Verification items for the finished model (mm, model axes). Face numbers are marked on the shaded views. A direction names the side the tool comes from. Coordinates: 2 decimals unless noted, no trailing zeros. Write each loop counter-clockwise with the first axis right and the second up, starting at its lowest first coordinate (ties: lowest second). Pieces come first, ordered by that corner, then holes. Notation, with made-up numbers: (-15, -21) -> (18, -21) arc R22 cw to (18, -4) -> close; hole circle Ø5 at (-35.5, 48.5). An arc over 180 degrees is marked (long way). Answer in a Markdown table with one row per item.
Autodesk Fusion 360 part; units mm, degrees
sketch "Çizim1" plane through (0, 0, 0) normal (0, 0, 1) x (1, 0, 0)
  line L0 (52.5, 65) -> (-52.5, 65)
  line L1 (-52.5, 65) -> (-52.5, -65)
  line L2 (-52.5, -65) -> (52.5, -65)
  line L3 (52.5, -65) -> (52.5, 65)
  line L4 (52.5, 65) -> (-52.5, -65) construction
  line L5 (-52.5, 65) -> (52.5, -65) construction
  dimension "d1" = 105
  dimension "d2" = 130
extrude "Ekstrüzyon1" add sketch "Çizim1" against normal blind 5
sketch "Çizim2" plane through (0, 0, 0) normal (0, 0, 1) x (-1, 0, 0)
  line L0 (-52.5, 65) -> (-52.5, -65)
  line L1 (-52.5, -65) -> (52.5, -65)
  line L2 (52.5, -65) -> (52.5, 65)
  line L3 (52.5, 65) -> (-52.5, 65)
  line L4 (47.5, 60) -> (-47.5, 60)
  line L5 (-47.5, 60) -> (-47.5, -60)
  line L6 (-47.5, -60) -> (47.5, -60)
  line L7 (47.5, -60) -> (47.5, 60)
  dimension "d5" = -5
extrude "Ekstrüzyon2" add sketch "Çizim2" along normal blind 30
extrude "Ekstrüzyon3" add 1 faces at (-47.5, 20, 10) along direction (1, 0, 0) blind 2.5
extrude "Ekstrüzyon4" add 1 faces at (47.5, -20, 10) along direction (-1, 0, 0) blind 2.5
extrude "Ekstrüzyon5" add 1 faces at (-50, 20, 30) along direction (0, 0, 1) blind 20
extrude "Ekstrüzyon6" add 1 faces at (-17.5, -65, 13.3333) along direction (0, -1, 0) blind 2
extrude "Ekstrüzyon7" add 1 faces at (-17.5, 65, 31.6667) along direction (0, 1, 0) blind 2
sketch "Çizim4" plane through (52.5, 0, 0) normal (1, 0, 0) x (0, 1, 0)
  line L0 (-67, -5) -> (67, -5)
  line L1 (67, -5) -> (67, 50)
  line L2 (67, 50) -> (-67, 50)
  line L3 (-67, 50) -> (-67, -5)
  circle A0 centre (-61, 40.25) radius 1.3
  line L4 (0, 50) -> (0, -5)
  circle A1 centre (61, 40.25) radius 1.3
  dimension "d18" = 2.6
  dimension "d19" = 9.75
  dimension "d20" = 6
extrude "Ekstrüzyon8" cut sketch "Çizim4" against normal blind 7.5 contours A0 | A1
extrude "Ekstrüzyon9" add 1 faces at (-15, 60, 29.8064) along direction (0, -1, 0) blind 5
extrude "Ekstrüzyon10" add 1 faces at (-15, -60, 29.8064) along direction (0, 1, 0) blind 5
mirror "Ayna1" about plane through (0, 0, 0) normal (1, 0, 0) of "Ekstrüzyon8"
sketch "Çizim5" plane through (-52.5, 0, 0) normal (-1, 0, 0) x (0, -1, 0)
  circle A0 centre (61, 40.25) radius 1.3
  circle A1 centre (-61, 40.25) radius 1.3
  line L0 (-67, -5) -> (67, -5)
  line L1 (67, -5) -> (67, 50)
  line L2 (67, 50) -> (-67, 50)
  line L3 (-67, 50) -> (-67, -5)
  line L4 (-55, 40) -> (-55, 25)
  line L5 (55, 40) -> (55, 25)
  line L6 (-55, 40) -> (55, 40)
  line L7 (55, 40) -> (55, 25)
  line L8 (55, 25) -> (-55, 25)
  line L9 (-55, 25) -> (-55, 40)
  dimension "d29" = 12
  dimension "d30" = 15
  dimension "d31" = 15
  dimension "d32" = 12
  dimension "d33" = 10
extrude "Ekstrüzyon11" cut sketch "Çizim5" against normal blind 105 contours L4 L5 L6 L7 L8 L9
sketch "Çizim6" plane through (-52.5, 0, 0) normal (-1, 0, 0) x (0, -1, 0)
  line L0 (55, 40) -> (55, 25)
  line L1 (55, 25) -> (-55, 25)
  line L2 (-55, 25) -> (-55, 40)
  line L3 (-55, 40) -> (55, 40)
  circle A0 centre (61, 40.25) radius 1.3
  circle A1 centre (-61, 40.25) radius 1.3
  line L4 (-67, -5) -> (67, -5)
  line L5 (67, -5) -> (67, 50)
  line L6 (67, 50) -> (-67, 50)
  line L7 (-67, 50) -> (-67, -5)
  line L8 (55, 25) -> (55, -5)
  line L9 (-55, 25) -> (-55, -5)
  line L10 (-55, 10) -> (55, 10)
  line L11 (-55, 20) -> (55, 20)
  line L12 (55, 20) -> (55, 0)
  line L13 (55, 0) -> (-55, 0)
  line L14 (-55, 0) -> (-55, 20)
extrude "Ekstrüzyon12" cut sketch "Çizim6" against normal blind 105 contours L8 L9 L10 L11 L12 L14 | L8 L9 L10 L12 L13 L14
sketch "Çizim7" plane through (0, 67, 0) normal (0, 1, 0) x (-1, 0, 0)
  line L0 (-52.5, 50) -> (-52.5, -5)
  line L1 (-52.5, -5) -> (52.5, -5)
  line L2 (52.5, -5) -> (52.5, 50)
  line L3 (52.5, 50) -> (-52.5, 50)
  line L4 (-45, 50) -> (-45, -5)
  line L5 (45, 50) -> (45, -5)
  line L6 (-45, 45) -> (45, 45)
  line L7 (45, 45) -> (45, 0)
  line L8 (45, 0) -> (-45, 0)
  line L9 (-45, 0) -> (-45, 45)
  dimension "d38" = 7.5
  dimension "d39" = 7.5
extrude "Ekstrüzyon13" cut sketch "Çizim7" against normal blind 134 contours L4 L5 L6 L7 L8 L9
sketch "Çizim8" plane through (0, 0, -5) normal (0, 0, -1) x (1, 0, 0)
  line L0 (52.5, -67) -> (52.5, 67)
  line L1 (52.5, 67) -> (-52.5, 67)
  line L2 (-52.5, 67) -> (-52.5, -67)
  line L3 (-52.5, -67) -> (52.5, -67)
  line L4 (5.5, -35.9) -> (-5.5, -35.9)
  line L5 (-5.5, -35.9) -> (-5.5, -56.1)
  line L6 (-5.5, -56.1) -> (5.5, -56.1)
  line L7 (5.5, -56.1) -> (5.5, -35.9)
  line L8 (0, -35.9) -> (0, -56.1)
  circle A0 centre (11.6, -31.8) radius 1.3
  circle A1 centre (11.6, -60.2) radius 1.3
  line L9 (11.6, -31.8) -> (11.6, -33.1)
  line L10 (11.6, -31.8) -> (11.6, -33.1)
  line L11 (11.6, -58.9) -> (11.6, -60.2)
  line L12 (11.6, -31.8) -> (11.6, -60.2)
  line L13 (11.6, -46) -> (5.5, -46)
  point P0 (5.5, -46)
  dimension "d42" = 11
  dimension "d43" = 20.2
  dimension "d44" = 10.9
  dimension "d45" = 28.4
  dimension "d46" = 2.6
  dimension "d47" = 2.6
  dimension "d48" = 6.1
extrude "Ekstrüzyon14" cut sketch "Çizim8" against normal blind 5 contours L4 L6 L7 L8 | A0 | A1 | L4 L5 L6 L8
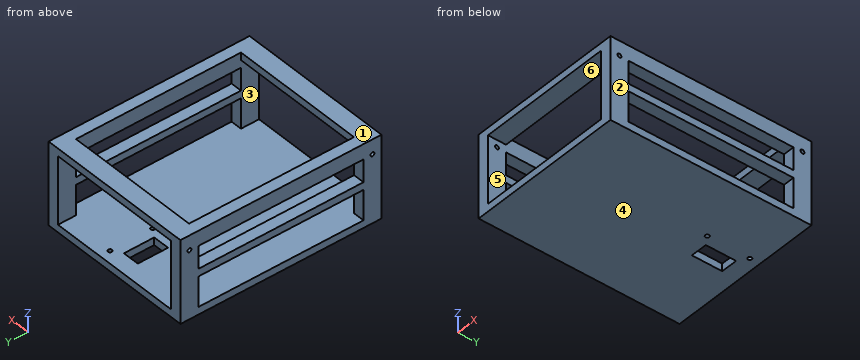
1. Depth check by flat-ended pin: P1, Ø4, axis at x = 27, y = 37.5, coming from the +Z side; P2, Ø3.5, axis at y = 61, z = 40.25, coming from the -X side. Enter the tip coordinate at first touch or a pass-through.
Geometry says:
| item | result |
|---|---|
| P1 | z = 0 |
| P2 | x = -52.5 |
2. Thickness scan on line 1 (X direction, y = -55.5, z = 36.5); line 2 (Y direction, x = 30, z = 46.5); line 3 (Z direction, x = 50, y = -61). Record the ranges inside material, lowest first. Write a range as from..to.
Geometry says:
| item | result |
|---|---|
| line 1 | -52.5..-45, 45..52.5 |
| line 2 | -67..-55, 55..67 |
| line 3 | -5..38.95, 41.55..50 |
3. Section check B-B, the plane x = 27. Record the boundary of the cut face in (y, z).
Geometry says:
| item | result |
|---|---|
| outline | (-67, -5) -> (67, -5) -> (67, 0) -> (-67, 0) -> close; (-67, 45) -> (-55, 45) -> (-55, 50) -> (-67, 50) -> close; (55, 45) -> (67, 45) -> (67, 50) -> (55, 50) -> close |
4. Section check C-C, the plane y = -40.5. Record the boundary of the cut face in (x, z), plus the area to 3 significant figures.
Geometry says:
| item | result |
|---|---|
| outline | (-52.5, -5) -> (52.5, -5) -> (52.5, 0) -> (-52.5, 0) -> close; (-52.5, 20) -> (-45, 20) -> (-45, 25) -> (-52.5, 25) -> close; (-52.5, 40) -> (-45, 40) -> (-45, 50) -> (-52.5, 50) -> close; (45, 20) -> (52.5, 20) -> (52.5, 25) -> (45, 25) -> close; (45, 40) -> (52.5, 40) -> (52.5, 50) -> (45, 50) -> close |
| area | 750 mm^2 |
5. Section check D-D, the plane x = 3.5. Record the boundary of the cut face in (y, z), plus the area to 3 significant figures.
Geometry says:
| item | result |
|---|---|
| outline | (-67, -5) -> (35.9, -5) -> (35.9, 0) -> (-67, 0) -> close; (-67, 45) -> (-55, 45) -> (-55, 50) -> (-67, 50) -> close; (55, 45) -> (67, 45) -> (67, 50) -> (55, 50) -> close; (56.1, -5) -> (67, -5) -> (67, 0) -> (56.1, 0) -> close |
| area | 689 mm^2 |
6. Tool access check on the marked faces 4, 5 and 6. Record the directions out of +Z, -Z, +X, -X, +Y, -Y that give a thin tool (end or side, any length) a straight path to the whole face; none if there is none.
Geometry says:
| item | result |
|---|---|
| face 4 | -Z, +X, -X, +Y, -Y |
| face 5 | none |
| face 6 | +Y, -Y |
7. Section check A-A, the plane z = 34. Record the boundary of the cut face in (x, y).
Geometry says:
| item | result |
|---|---|
| outline | (-52.5, -67) -> (-45, -67) -> (-45, -55) -> (-52.5, -55) -> close; (-52.5, 55) -> (-45, 55) -> (-45, 67) -> (-52.5, 67) -> close; (45, -67) -> (52.5, -67) -> (52.5, -55) -> (45, -55) -> close; (45, 55) -> (52.5, 55) -> (52.5, 67) -> (45, 67) -> close |
8. Mould release check, pull along Z, two halves, no side actions. Record for the marked faces 1, 2 and 3: released by +Z, released by -Z, zero draft, split by the parting line, or undercut.
Geometry says:
| item | result |
|---|---|
| face 1 | released by +Z |
| face 2 | zero draft |
| face 3 | undercut |
